Source: CAD feature listing. Evaluate the final solid. Frame: model axes, mm. A direction names the side the tool comes from. Give positions to 0.01 mm unless a question says otherwise; leave off trailing zeros. Order: outer loops, then holes, each group sorted by start corner. A loop starts at its lowest first (then second) coordinate and runs counter-clockwise, first axis right, second up.
from build123d import *

# Parameters (mm, degrees)
F1_DEPTH = 3
F3_DEPTH = 3
F4_R     = 1.5


with BuildPart() as f1:
    # F0 (on Top) → F1 (new body)
    with BuildSketch(Plane.XY):
        with BuildLine():
            ThreePointArc((9, 0), (0, -9), (-9, 0))
            Line((-9, 0), (-9, 40))
            Line((-9, 40), (-23, 40))
            Line((-23, 40), (-23, -5))
            ThreePointArc((-23, -5), (-20.5, -7.5), (-18, -5))
            Line((-18, -5), (-18, 35))
            ThreePointArc((-18, 35), (-15, 36.8), (-12, 35))
            Line((-12, 35), (-12, 0))
            ThreePointArc((-12, 0), (0, -12), (12, 0))
            Line((12, 0), (12, 33))
            ThreePointArc((12, 33), (10.5, 34.5), (9, 33))
            Line((9, 33), (9, 0))
        make_face()
    extrude(amount=F1_DEPTH)

    # F2 (on face) → F3 (join)
    with BuildSketch(Plane.XY.offset(3)):
        with BuildLine():
            Line((-18, -5), (-18, 32))
            ThreePointArc((-18, 32), (-20.5, 34.5), (-23, 32))
            Line((-23, 32), (-23, -5))
            ThreePointArc((-23, -5), (-20.5, -7.5), (-18, -5))
        make_face()
    extrude(amount=F3_DEPTH)

    # F4
    f4_edges = [f1.edges().sort_by_distance(p)[0] for p in [
        (-23, 40, 1.5),
        (-9, 40, 1.5),
    ]]
    fillet(f4_edges, radius=F4_R)


solid = f1.part
(1) Line query: line 1 along X through (y, z) = (25.5, 1.45); line 2 along X through (y, z) = (33.5, 0.95); line 3 along X through (y, z) = (8, 3.6). Output: solid intervals per line, ascending.
(2) Access query for faces 1 (the cylindrical face through (-20.4, 34.5, 4.5)), 2 (the flat face through (-21, 14, 6)), 3 (the flat face through (9, 17, 1)), 4 (the flat face through (-12, 18, 1)), 5 (the flat face through (12, 16, 1)). Directions: +Z, -Z, +X, -X, +Y, -Y. A direction counts if a zero-diameter tool reaches every point of the face in a straight line with its end or side. Return the directions, or none.
(3) Section A-A, the plane y = 28.5. Return loops of the section in (x, z).
(4) Section B-B, the plane x = -20.5. Return loops of the section in (y, z), plus the area to 4 significant figures.
(5) Pin query (flat end, axial travel): pin 1 Ø2 at (y, z) = (-6.5, 2) entering from -X; pin 2 Ø3 at (x, z) = (-5.5, 3) entering from -Y; pin 3 Ø8 at (x, y) = (8.5, 12) entering from -Z; pin 4 Ø2 at (x, z) = (-16.5, 2.5) entering from -Y. Return the tip coordinate at first contact, or that it passes through.
(6) Section D-D, the plane y = -3. Return loops of the section in (x, z).
(7) Section C-C, the plane z = 3.7. Return loops of the section in (x, y), plus the area to 3 significant figures.
Checks:
1. line 1: x = -23 to -18, -12 to -9, 9 to 12
1. line 2: x = -23 to -18, -12 to -9, 9.09 to 11.91
1. line 3: x = -23 to -18
2. face 1: +Z, +Y
2. face 2: +Z, +X, -X, +Y, -Y
2. face 3: +Z, -Z, +Y
2. face 4: +Z, -Z, -Y
2. face 5: +Z, -Z, +X, +Y, -Y
3. outline: (-23, 0) - (-18, 0) - (-18, 6) - (-23, 6) - close; (-12, 0) - (-9, 0) - (-9, 3) - (-12, 3) - close; (9, 0) - (12, 0) - (12, 3) - (9, 3) - close
4. outline: (-7.5, 0) - (40, 0) - (40, 3) - (34.5, 3) - (34.5, 6) - (-7.5, 6) - close
4. area: 268.5 mm2
5. pin 1: stops at x = -22.95
5. pin 2: stops at y = -11.31
5. pin 3: stops at z = 0
5. pin 4: stops at y = 35.7
6. outline: (-23, 0) - (-18, 0) - (-18, 6) - (-23, 6) - close; (-11.62, 0) - (-8.49, 0) - (-8.49, 3) - (-11.62, 3) - close; (8.49, 0) - (11.62, 0) - (11.62, 3) - (8.49, 3) - close
7. outline: (-23, -5) arc R2.5 ccw to (-18, -5) - (-18, 32) arc R2.5 ccw to (-23, 32) - close
7. area: 205 mm2
